from build123d import *

# Parameters (mm, degrees)
BOSS_EXTRUDE1_DEPTH = 6
SKETCH3_R           = 6.5
BOSS_EXTRUDE2_DEPTH = 10
CUT_EXTRUDE7_DEPTH  = 9
CIRPATTERN1_COUNT   = 4
SKETCH12_R          = 6.5
CUT_EXTRUDE8_DEPTH  = 30


with BuildPart() as part:
    # Sketch1 → Boss-Extrude1 (new body)
    with BuildSketch(Plane.XY):
        with BuildLine():
            Line((-5.05, 9.05), (5.05, 9.05))
            ThreePointArc((5.05, 9.05), (7.878427125, 7.878427125), (9.05, 5.05))
            Line((9.05, 5.05), (9.05, -5.05))
            ThreePointArc((9.05, -5.05), (7.878427125, -7.878427125), (5.05, -9.05))
            Line((5.05, -9.05), (-5.05, -9.05))
            ThreePointArc((-5.05, -9.05), (-7.878427125, -7.878427125), (-9.05, -5.05))
            Line((-9.05, -5.05), (-9.05, 5.05))
            ThreePointArc((-9.05, 5.05), (-7.878427125, 7.878427125), (-5.05, 9.05))
        make_face()
    extrude(amount=BOSS_EXTRUDE1_DEPTH)

    # Sketch3 → Boss-Extrude2 (add)
    with BuildSketch(Plane.XY.offset(6)):
        Polygon((-5, -7), (5, -7), (7, -5), (7, 5), (5, 7), (-5, 7), (-7, 5), (-7, -5), align=None)
        Circle(SKETCH3_R, mode=Mode.SUBTRACT)
    extrude(amount=BOSS_EXTRUDE2_DEPTH)

    # Sketch11 → Cut-Extrude7 (cut)
    with BuildSketch(Plane.XY.offset(16)):
        Polygon((0, 0), (7, 0.45), (7, -0.45), align=None)
    cut_extrude7 = extrude(amount=-CUT_EXTRUDE7_DEPTH, mode=Mode.SUBTRACT)

    # CirPattern1: Cut-Extrude7 ×4 about axis
    cirpattern1_axis = Axis((0, 0, 16), (0, 0, -1))
    for i in range(1, CIRPATTERN1_COUNT):
        add(cut_extrude7.rotate(cirpattern1_axis, i * 360 / CIRPATTERN1_COUNT), mode=Mode.SUBTRACT)

    # Sketch12 → Cut-Extrude8 (cut)
    with BuildSketch(Plane.XY.offset(6)):
        with Locations(Location((0, 0.192488852, 0), (0, 0, 359.151599859))):
            Circle(SKETCH12_R)
    extrude(amount=-CUT_EXTRUDE8_DEPTH, mode=Mode.SUBTRACT)


solid = part.part
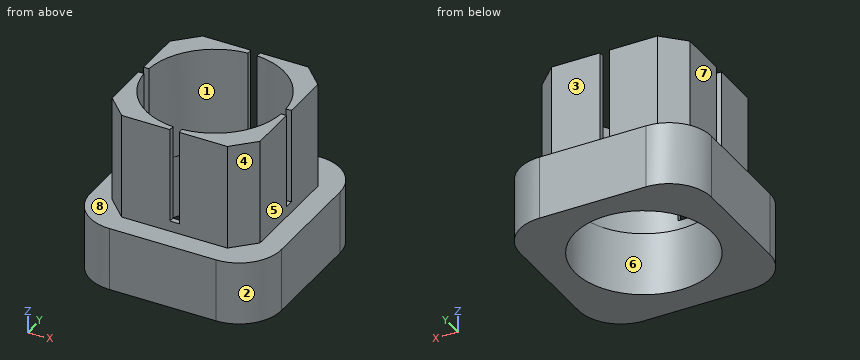
Design review of the part built by this model. Coordinates are the model's own, in mm. Face numbers are marked on the shaded views. A direction names the side the tool comes from. Coordinates: 2 decimals unless noted, no trailing zeros. Loops run counter-clockwise (first coordinate to the right, second up) from the corner with the lowest first, then second, coordinate; pieces in that order, holes last. Notation, with made-up numbers: (83.5, -16) - (91.5, -16) arc R14 ccw to (91.5, 8) - close; hole circle Ø9 at (-9, -40). An arc over 180 degrees is marked (long way). Use CSV: the item, a comma, the result in double quotes. Start each with the question number.
1. Add section A-A on z = 14.75. Give the boundary of the cut face in (x, y), plus the area to 3 significant figures.
2. Add section C-C on y = -5.5. Give the boundary of the cut face in (x, z), plus the area to 3 significant figures.
3. For the marked faces 4, 5, 6, 7 and 8, list the 3-axis set-ups (+Z, -Z, +X, -X, +Y, -Y) from which the entire face can be reached by the end or side of a thin tool; tool diameter is ignored.
4. Clearance check with flat-ended pins moving along their axes: pin 1 (5 mm diameter, centred on x = -1, z = 10, fed in from +Y); pin 2 (3 mm diameter, centred on y = -2.5, z = 11, fed in from -X); pin 3 (0.6 mm diameter, centred on x = 6.5, y = 0, fed in from +Z). State where each tip first meets the part, or that it passes through.
5. Add section B-B on x = 0. Give the boundary of the cut face in (y, z), plus the area to 3 significant figures.
6. To check wall thickness, follow probe 1 along Y at (x, z) = (0, 3.2); probe 2 along Y at (x, z) = (5, 2.75); probe 3 along Z at (x, y) = (-3.75, 7.5). State the ranges of each line that lie inside material, in increasing order.
7. Add section D-D on z = 2.5. Give the boundary of the cut face in (x, y), plus the area to 3 significant figures.
8. Mouldability with a two-part tool opening along Y and no side actions: class the marked faces 1, 2 and 3 as released by +Y, released by -Y, zero draft, split by the parting line, or undercut.
Resolved:
1,outline,"(-7, -5) - (-5, -7) - (-0.45, -7) - (-0.42, -6.49) arc R6.5 cw to (-6.49, -0.42) - (-7, -0.45) - close; (-7, 0.45) - (-6.49, 0.42) arc R6.5 cw to (-0.42, 6.49) - (-0.45, 7) - (-5, 7) - (-7, 5) - close; (0.42, -6.49) - (0.45, -7) - (5, -7) - (7, -5) - (7, -0.45) - (6.49, -0.42) arc R6.5 cw to start; (0.42, 6.49) arc R6.5 cw to (6.49, 0.42) - (7, 0.45) - (7, 5) - (5, 7) - (0.45, 7) - close"
1,area,"53.5 mm2"
2,outline,"(-9.02, 0) - (-3.14, 0) - (-3.14, 6) - (-3.46, 6) - (-3.46, 16) - (-6.5, 16) - (-6.5, 6) - (-9.02, 6) - close; (3.14, 0) - (9.02, 0) - (9.02, 6) - (6.5, 6) - (6.5, 16) - (3.46, 16) - (3.46, 6) - (3.14, 6) - close"
2,area,"131 mm2"
3,face 4,"+Z, +X, -Y"
3,face 5,"+Z, +X, +Y, -Y"
3,face 6,"-Z"
3,face 7,"+Z, -X, +Y, -Y"
3,face 8,"+Z"
4,pin 1,"y = 7"
4,pin 2,"x = -7"
4,pin 3,"z = 7"
5,outline,"(-9.05, 0) - (-6.31, 0) - (-6.31, 6) - (-6.5, 6) - (-6.5, 7) - (-7, 7) - (-7, 6) - (-9.05, 6) - close; (6.5, 6) - (6.69, 6) - (6.69, 0) - (9.05, 0) - (9.05, 6) - (7, 6) - (7, 7) - (6.5, 7) - close"
5,area,"31.6 mm2"
6,probe 1,"-9.05 to -6.31, 6.69 to 9.05"
6,probe 2,"-9.05 to -3.96, 4.35 to 9.05"
6,probe 3,"0 to 6"
7,outline,"(-9.05, -5.05) arc R4 ccw to (-5.05, -9.05) - (5.05, -9.05) arc R4 ccw to (9.05, -5.05) - (9.05, 5.05) arc R4 ccw to (5.05, 9.05) - (-5.05, 9.05) arc R4 ccw to (-9.05, 5.05) - close; hole circle Ø13 at (0, 0.19)"
7,area,"181 mm2"
8,face 1,"undercut"
8,face 2,"released by -Y"
8,face 3,"released by +Y"
